```python
from build123d import *

# Parameters (mm, degrees)
SKETCH_1_R          = 100
EXTRUDE_1_DEPTH     = 5
SKETCH_3_R          = 3
CUT_EXTRUDE_1_DEPTH = 142.509716981
SKETCH_5_R          = 1.5
CUT_EXTRUDE_2_DEPTH = 142.509716981
SKETCH_6_R          = 12
CUT_EXTRUDE_3_DEPTH = 142.509716981
EXTRUDE_2_DEPTH     = 57
SKETCH_9_R          = 100
SKETCH_9_R_2        = 30
EXTRUDE_4_DEPTH     = 15
SKETCH_10_R         = 43
CUT_EXTRUDE_4_DEPTH = 11


with BuildPart() as part:
    # 草图1 → 凸台-拉伸1 (new body)
    with BuildSketch(Plane(origin=(0, 0, 0), x_dir=(1, 0, 0), z_dir=(0, 1, 0))):
        with Locations(Location((0, 0, 0), (0, 0, 270))):
            Circle(SKETCH_1_R)
    extrude(amount=EXTRUDE_1_DEPTH)

    # 草图3 → 切除-拉伸1 (cut, through all)
    with BuildSketch(Plane.XZ):
        with Locations(Location((0, 90, 0), (0, 0, 270))):
            Circle(SKETCH_3_R)
        with Locations(Location((90, 0, 0), (0, 0, 270))):
            Circle(SKETCH_3_R)
        with Locations(Location((0, -90, 0), (0, 0, 270))):
            Circle(SKETCH_3_R)
        with Locations(Location((-90, 0, 0), (0, 0, 270))):
            Circle(SKETCH_3_R)
    extrude(amount=-CUT_EXTRUDE_1_DEPTH, mode=Mode.SUBTRACT)

    # 草图5 → 切除-拉伸2 (cut, through all)
    with BuildSketch(Plane(origin=(0, 5, 0), x_dir=(1, 0, 0), z_dir=(0, 1, 0))):
        with Locations(Location((-15.5, 15.5, 0), (0, 0, 270))):
            Circle(SKETCH_5_R)
        with Locations(Location((15.5, 15.5, 0), (0, 0, 270))):
            Circle(SKETCH_5_R)
        with Locations(Location((-15.5, -15.5, 0), (0, 0, 270))):
            Circle(SKETCH_5_R)
        with Locations(Location((15.5, -15.5, 0), (0, 0, 270))):
            Circle(SKETCH_5_R)
    extrude(amount=-CUT_EXTRUDE_2_DEPTH, mode=Mode.SUBTRACT)

    # 草图6 → 切除-拉伸3 (cut, through all)
    with BuildSketch(Plane(origin=(0, 5, 0), x_dir=(1, 0, 0), z_dir=(0, 1, 0))):
        with Locations(Location((0, 0, 0), (0, 0, 270))):
            Circle(SKETCH_6_R)
    extrude(amount=-CUT_EXTRUDE_3_DEPTH, mode=Mode.SUBTRACT)

    # 草图7 → 凸台-拉伸2 (add)
    with BuildSketch(Plane(origin=(0, 5, 0), x_dir=(1, 0, 0), z_dir=(0, 1, 0))):
        Polygon((-50.809093778, 57.317929583), (-37.568542495, 57.317929583), (-36.568542495, 56.317929583), (-36.568542495, 54.317929583), (-37.568542495, 53.317929583), (-46.809093778, 53.317929583), (-51.809093778, 48.317929583), (-51.809093778, 38.348523411), (-52.809093778, 37.348523411), (-54.809093778, 37.348523411), (-55.809093778, 38.348523411), (-55.809093778, 52.317929583), align=None)
        Polygon((-55.809093778, -52.317929583), (-55.809093778, -36.788561579), (-54.809093778, -35.788561579), (-52.809093778, -35.788561579), (-51.809093778, -36.788561579), (-51.809093778, -48.317929583), (-46.809093778, -53.317929583), (-36.809093778, -53.317929583), (-35.809093778, -54.317929583), (-35.809093778, -56.317929583), (-36.809093778, -57.317929583), (-50.809093778, -57.317929583), align=None)
        Polygon((55.809093778, -52.317929583), (55.809093778, -37.390513406), (54.809093778, -36.390513406), (52.809093778, -36.390513406), (51.809093778, -37.390513406), (51.809093778, -48.317929583), (46.809093778, -53.317929583), (38.327991212, -53.317929583), (37.327991212, -54.317929583), (37.327991212, -56.317929583), (38.327991212, -57.317929583), (50.809093778, -57.317929583), align=None)
        Polygon((50.809093778, 57.317929583), (37.568542495, 57.317929583), (36.568542495, 56.317929583), (36.568542495, 54.317929583), (37.568542495, 53.317929583), (46.809093778, 53.317929583), (51.809093778, 48.317929583), (51.809093778, 39.097910499), (52.809093778, 38.097910499), (54.809093778, 38.097910499), (55.809093778, 39.097910499), (55.809093778, 52.317929583), align=None)
    extrude(amount=-EXTRUDE_2_DEPTH)

    # 草图9 → 凸台-拉伸4 (add)
    with BuildSketch(Plane(origin=(0, 5, 0), x_dir=(1, 0, 0), z_dir=(0, 1, 0))):
        with Locations(Location((0, 0, 0), (0, 0, 270))):
            Circle(SKETCH_9_R)
        with Locations(Location((0, 0, 0), (0, 0, 270))):
            Circle(SKETCH_9_R_2, mode=Mode.SUBTRACT)
    extrude(amount=EXTRUDE_4_DEPTH)

    # 草图10 → 切除-拉伸4 (cut)
    with BuildSketch(Plane(origin=(0, 20, 0), x_dir=(1, 0, 0), z_dir=(0, 1, 0))):
        with Locations(Location((0, 0, 0), (0, 0, 270))):
            Circle(SKETCH_10_R)
    extrude(amount=-CUT_EXTRUDE_4_DEPTH, mode=Mode.SUBTRACT)


solid = part.part
```
Check sheet for the modelled part. Datum: model origin and axes. Units: mm. A direction names the side the tool comes from. Coordinates: 2 decimals unless noted, no trailing zeros. Order: outer loops, then holes, each group sorted by start corner. A loop starts at its lowest first (then second) coordinate and runs counter-clockwise, first axis right, second up. Notation, with made-up numbers: M 36.25,23.25 L 91.25,23.25 A13 ccw 91.25,43.25 Z; hole C 68,-27 d3. An arc over 180 degrees is marked long. One line per question, with ' | ' between items. Start each with the question number.
Item 1: Mould release check, pull along X, two halves, no side actions. Record for faces 6 (the flat face through (44, -26, 57.318)), 7 (the flat face through (53.344, -25.636, -54.783)), 8 (the flat face through (0, 5, 90)), 9 (the flat face through (-49.274, -25.636, -50.853)): pulls with the +X half, pulls with the -X half, needs draft (parallel to the pull), parting line crosses it, or undercut.
Item 2: Access from +Z, -Z, +X, -X, +Y, -Y to the whole of each face (thin tool, end or side, straight path). Record for faces 1 (the flat face through (50, -52, -52)), 2 (the cylindrical face through (0, 2, -87)), 3 (the cylindrical face through (29.061, 14.577, -31.693)), 4 (the flat face through (-44, -26, 57.318)), 5 (the flat face through (-44, -26, -57.318)).
Item 3: Sectioned sample at B-B on x = 0. Record the cut outline in (y, z).
Item 4: Sectioned sample at A-A on z = 0. Record the cut outline in (x, y), and give its area (3 significant figures).
Item 5: Sectioned sample at C-C on y = 12.5. Record the cut outline in (x, z), and give its area (3 significant figures).
Item 6: Material ranges on line 1 (X direction, y = 1.65, z = 0); line 2 (X direction, y = 6.5, z = 0); line 3 (Y direction, x = 68, z = 21.5), recorded low to high.
Item 7: Gauge pin test, flat ends, axial feed: P1, Ø8, axis at y = -38, z = -43, coming from the +X side; P2, Ø3, axis at x = -44.5, y = -38, coming from the +Z side; P3, Ø8, axis at x = 56, y = -21, coming from the +Z side; P4, Ø2.5, axis at x = -15.5, z = -15.5, coming from the +Y side. Record the tip position at first contact, or that the pin passes through.
Item 8: Sectioned sample at D-D on z = -20.5. Record the cut outline in (x, y).
Answer below:
1) face 6: needs draft | face 7: pulls with the +X half | face 8: undercut | face 9: undercut
2) face 1: +Z, -Z, +X, -X, -Y | face 2: -Y | face 3: +Y | face 4: +Z, +X, -X, -Y | face 5: -Z, +X, -X, -Y
3) outline: M 0,-100 L 20,-100 L 20,-43 L 9,-43 L 9,-30 L 5,-30 L 5,-12 L 0,-12 L 0,-87 L 5,-87 L 5,-93 L 0,-93 Z; M 0,12 L 5,12 L 5,30 L 9,30 L 9,43 L 20,43 L 20,100 L 0,100 L 0,93 L 5,93 L 5,87 L 0,87 Z
4) outline: M -100,0 L -93,0 L -93,5 L -87,5 L -87,0 L -12,0 L -12,5 L -30,5 L -30,9 L -43,9 L -43,20 L -100,20 Z; M 12,0 L 87,0 L 87,5 L 93,5 L 93,0 L 100,0 L 100,20 L 43,20 L 43,9 L 30,9 L 30,5 L 12,5 Z | area: 2,630 mm^2
5) outline: C 0,0 d200; hole C 0,0 d86 | area: 25,600 mm^2
6) line 1: x = -100 to -93, -87 to -12, 12 to 87, 93 to 100 | line 2: x = -100 to -30, 30 to 100 | line 3: y = 0 to 20
7) P1: stops at x = 55.81 | P2: stops at z = 57.32 | P3: stops at z = 56.13 | P4: passes through
8) outline: M -97.88,0 L 97.88,0 L 97.88,20 L 37.8,20 L 37.8,9 L 21.9,9 L 21.9,5 L -21.9,5 L -21.9,9 L -37.8,9 L -37.8,20 L -97.88,20 Z
